```python
from build123d import *

# Parameters (mm, degrees)
ESQUISSE1_W             = 15
ESQUISSE1_H             = 13
BOSS_EXTRU_1_DEPTH      = 10
CONG_1_R                = 1
ESQUISSE2_W             = 17.6
ESQUISSE2_H             = 10.6
ENL_V_MAT_EXTRU_1_DEPTH = 1
CONG_2_R                = 1
CONG_2_OF_SYM_TRIE1_R   = 1
ESQUISSE3_R             = 3
BOSS_EXTRU_2_DEPTH      = 8


with BuildPart() as part:
    # Esquisse1 → Boss.-Extru.1 (new, symmetric)
    with BuildSketch(Plane.XY):
        Rectangle(ESQUISSE1_W, ESQUISSE1_H)
    extrude(amount=BOSS_EXTRU_1_DEPTH, both=True)

    # Congé1
    cong_1_edges = [part.edges().sort_by_distance(p)[0] for p in [
        (0, 6.5, -10),
        (0, -6.5, -10),
    ]]
    fillet(cong_1_edges, radius=CONG_1_R)

    # Esquisse2 → Enlèv. mat.-Extru.1 (cut)
    with BuildSketch(Plane(origin=(7.5, 0, 0), x_dir=(0, 0, -1), z_dir=(1, 0, 0))):
        Rectangle(ESQUISSE2_W, ESQUISSE2_H)
    enl_v_mat_extru_1 = extrude(amount=-ENL_V_MAT_EXTRU_1_DEPTH, mode=Mode.SUBTRACT)

    # Congé2
    cong_2_edges = [part.edges().sort_by_distance(p)[0] for p in [
        (7, 5.3, -8.8),
        (7, -5.3, -8.8),
    ]]
    fillet(cong_2_edges, radius=CONG_2_R)

    # Symétrie1: Enlèv. mat.-Extru.1 across plane
    add(enl_v_mat_extru_1.mirror(Plane(origin=(0, 0, 0), x_dir=(0, 0, 1), z_dir=(1, 0, 0))), mode=Mode.SUBTRACT)

    # Congé2 of Symétrie1
    cong_2_of_sym_trie1_edges = [part.edges().sort_by_distance(p)[0] for p in [
        (-7, 5.3, -8.8),
        (-7, -5.3, -8.8),
    ]]
    fillet(cong_2_of_sym_trie1_edges, radius=CONG_2_OF_SYM_TRIE1_R)

    # Esquisse3 → Boss.-Extru.2 (add)
    with BuildSketch(Plane.XY.offset(10)):
        Circle(ESQUISSE3_R)
    extrude(amount=BOSS_EXTRU_2_DEPTH)


solid = part.part
```
Model file for the job. Use its own axes, mm. A direction names the side the tool comes from. Coordinates: 2 decimals unless noted, no trailing zeros. Write each loop counter-clockwise with the first axis right and the second up, starting at its lowest first coordinate (ties: lowest second). Pieces come first, ordered by that corner, then holes. Notation, with made-up numbers: (53, 54) - (80, 54) arc R33 cw to (80, 92) - close; hole circle Ø3 at (-26.5, -18). An arc over 180 degrees is marked (long way). One line per question, with ' | ' between items. Start each with the question number.
Q1. Pull direction Z, two halves, no side cores. Call faces 1 (the face through (0, 0, 18)), 2 (the face through (-7, -5.3, 1)), 3 (the face through (0, 6.5, 1)): pulls with the +Z half, pulls with the -Z half, needs draft (parallel to the pull), parting line crosses it, or undercut.
Q2. 3-axis set-ups, long thin cutter, end or side, ignore diameter. For faces 4 (the face through (6.993, -5.015, -8.499)), 5 (the face through (0, -6.5, 1)), 6 (the face through (0.105, -6.199, -9.715)), 7 (the face through (-3, 0, 14)), 8 (the face through (-6.5, 0, 0)): which of +Z, -Z, +X, -X, +Y, -Y reach the whole face in a straight line?
Q3. Drill centre lines: line 1 (Y direction, x = 7.25, z = 4.75); line 2 (Z direction, x = 4, y = 0.5); line 3 (X direction, y = -1, z = 2). Where is each one in solid material? Low to high. Write a range as [from, to].
Q4. Cut at D-D, the plane x = -4.75. List the corners of the cut face in (y, z), then the cut area to 3 significant figures.
Q5. Cut at C-C, the plane x = 0. List the corners of the cut face in (y, z).
Q6. Cut at A-A, the plane y = 0. List the corners of the cut face in (x, z).
Q7. Pin check, flat tips, straight feed: pin 1 (5 mm diameter, centred on y = -0.5, z = -2, fed in from -X); pin 2 (1.5 mm diameter, centred on y = -3, z = 7.5, fed in from +X); pin 3 (0.8 mm diameter, centred on x = -7, y = -2, fed in from +Z). Stop position of each tip, or through.
Q8. Cut at B-B, the plane z = 0.5. List the corners of the cut face in (x, y), then the cut area to 3 significant figures.
Answer below:
1) face 1: pulls with the +Z half | face 2: undercut | face 3: needs draft
2) face 4: +X | face 5: +Z, -Z, +X, -X, -Y | face 6: -Z, +X, -X, -Y | face 7: +Z | face 8: -X
3) line 1: [-6.5, -5.3], [5.3, 6.5] | line 2: [-10, 10] | line 3: [-6.5, 6.5]
4) outline: (-6.5, -9) arc R1 ccw to (-5.5, -10) - (5.5, -10) arc R1 ccw to (6.5, -9) - (6.5, 10) - (-6.5, 10) - close | area: 260 mm^2
5) outline: (-6.5, -9) arc R1 ccw to (-5.5, -10) - (5.5, -10) arc R1 ccw to (6.5, -9) - (6.5, 10) - (3, 10) - (3, 18) - (-3, 18) - (-3, 10) - (-6.5, 10) - close
6) outline: (-7.5, -10) - (7.5, -10) - (7.5, -8.8) - (6.5, -8.8) - (6.5, 8.8) - (7.5, 8.8) - (7.5, 10) - (3, 10) - (3, 18) - (-3, 18) - (-3, 10) - (-7.5, 10) - (-7.5, 8.8) - (-6.5, 8.8) - (-6.5, -8.8) - (-7.5, -8.8) - close
7) pin 1: x = -6.5 | pin 2: x = 6.5 | pin 3: z = 10
8) outline: (-7.5, -6.5) - (7.5, -6.5) - (7.5, -5.3) - (6.5, -5.3) - (6.5, 5.3) - (7.5, 5.3) - (7.5, 6.5) - (-7.5, 6.5) - (-7.5, 5.3) - (-6.5, 5.3) - (-6.5, -5.3) - (-7.5, -5.3) - close | area: 174 mm^2
